Geometry: final body of the model. Coordinates: model frame, mm. Face numbers are marked on the shaded views. A direction names the side the tool comes from. Coordinates: 2 decimals unless noted, no trailing zeros. Write each loop counter-clockwise with the first axis right and the second up, starting at its lowest first coordinate (ties: lowest second). Pieces come first, ordered by that corner, then holes. Notation, with made-up numbers: (33.5, 13) -> (47.5, 13) arc R12 ccw to (47.5, 30) -> close; hole circle Ø10 at (17.25, 54). An arc over 180 degrees is marked (long way). One line per item, written item: value.
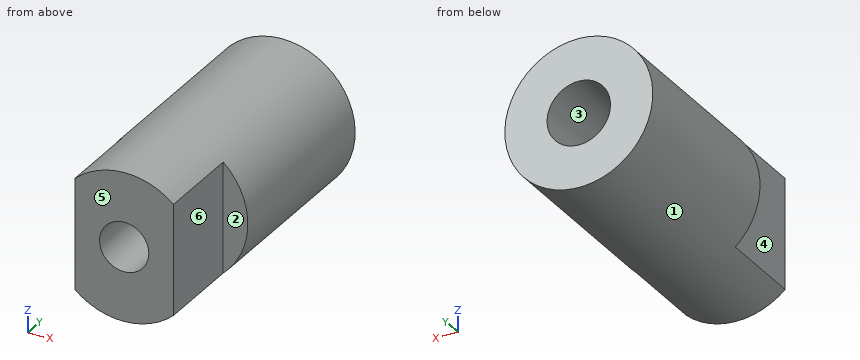
```python
from build123d import *

# Parameters (mm, degrees)
SKETCH1_R                  = 10.5
BOSS_EXTRUDE1_DEPTH        = 40.1
M10X1_0_TAPPED_HOLE1_D     = 9
M10X1_0_TAPPED_HOLE1_DEPTH = 23
M10X1_0_TAPPED_HOLE1_TIP   = 2.703872786
M8X1_0_TAPPED_HOLE1_D      = 7
M8X1_0_TAPPED_HOLE1_DEPTH  = 19
M8X1_0_TAPPED_HOLE1_TIP    = 2.103012167
CUT_EXTRUDE1_DEPTH         = 43.761080435
CUT_EXTRUDE1_DEPTH_BACK    = 43.761080435
SKETCH6_W                  = 3.5
SKETCH6_H                  = 12.7


with BuildPart() as part:
    # Sketch1 → Boss-Extrude1 (new body)
    with BuildSketch(Plane(origin=(0, 0, 0), x_dir=(1, 0, 0), z_dir=(0, 1, 0))):
        with Locations(Location((0, 0, 0), (0, 0, 270))):
            Circle(SKETCH1_R)
    extrude(amount=BOSS_EXTRUDE1_DEPTH)

    # M10x1.0 Tapped Hole1
    with Locations(Plane(origin=(0, 40.1, 0), x_dir=(1, 0, 0), z_dir=(0, 1, 0))):
        with Locations((0, 0)):
            Hole(M10X1_0_TAPPED_HOLE1_D / 2, depth=M10X1_0_TAPPED_HOLE1_DEPTH)
            with Locations((0, 0, -(M10X1_0_TAPPED_HOLE1_DEPTH + M10X1_0_TAPPED_HOLE1_TIP / 2))):  # 118° drill point
                Cone(0, M10X1_0_TAPPED_HOLE1_D / 2, M10X1_0_TAPPED_HOLE1_TIP, mode=Mode.SUBTRACT)

    # M8x1.0 Tapped Hole1
    with Locations(Plane(origin=(0, 0, 0), x_dir=(-1, 0, 0), z_dir=(0, -1, 0))):
        with Locations((0, 0)):
            Hole(M8X1_0_TAPPED_HOLE1_D / 2, depth=M8X1_0_TAPPED_HOLE1_DEPTH)
            with Locations((0, 0, -(M8X1_0_TAPPED_HOLE1_DEPTH + M8X1_0_TAPPED_HOLE1_TIP / 2))):  # 118° drill point
                Cone(0, M8X1_0_TAPPED_HOLE1_D / 2, M8X1_0_TAPPED_HOLE1_TIP, mode=Mode.SUBTRACT)

    # Sketch6 → Cut-Extrude1 (cut, two sides: drawn at the far end of the back side and taken through both)
    with BuildSketch(Plane.XY.offset(-CUT_EXTRUDE1_DEPTH_BACK)):
        with Locations((-8.75, 6.35)):
            Rectangle(SKETCH6_W, SKETCH6_H)
        with Locations((8.75, 6.35)):
            Rectangle(SKETCH6_W, SKETCH6_H)
    extrude(amount=CUT_EXTRUDE1_DEPTH + CUT_EXTRUDE1_DEPTH_BACK, mode=Mode.SUBTRACT)


solid = part.part
```
(1) Section B-B (x = 0). Return the cut outline in (y, z).
Responses:
outline: (0, -10.5) -> (40.1, -10.5) -> (40.1, -4.5) -> (17.1, -4.5) -> (16.5, -3.5) -> (0, -3.5) -> close; (0, 3.5) -> (16.5, 3.5) -> (17.1, 4.5) -> (40.1, 4.5) -> (40.1, 10.5) -> (0, 10.5) -> close
(2) Section C-C (y = 5). Return the cut outline in (x, z), then the cut area to 3 significant figures.
Responses:
outline: (-7, -7.83) arc R10.5 ccw to (7, -7.83) -> (7, 7.83) arc R10.5 ccw to (-7, 7.83) -> close; hole circle Ø7 at (0, 0)
area: 232 mm2
(3) Section D-D (z = -5.5). Return the cut outline in (x, y), then the cut area to 3 significant figures.
Responses:
outline: (-8.94, 12.7) -> (-7, 12.7) -> (-7, 0) -> (7, 0) -> (7, 12.7) -> (8.94, 12.7) -> (8.94, 40.1) -> (-8.94, 40.1) -> close
area: 668 mm2
(4) Pull-direction query (Z, two-part tool) for the marked faces 1, 2 and 3; classes: released by +Z, released by -Z, zero draft, split by the parting line, or undercut.
Responses:
face 1: split by the parting line
face 2: zero draft
face 3: undercut
(5) Section A-A (z = 0). Return the cut outline in (x, y).
Responses:
outline: (-10.5, 12.7) -> (-7, 12.7) -> (-7, 0) -> (-3.5, 0) -> (-3.5, 16.5) -> (-4.5, 17.1) -> (-4.5, 40.1) -> (-10.5, 40.1) -> close; (3.5, 0) -> (7, 0) -> (7, 12.7) -> (10.5, 12.7) -> (10.5, 40.1) -> (4.5, 40.1) -> (4.5, 17.1) -> (3.5, 16.5) -> close
(6) First-contact query: pin 1 (5.5 mm diameter, centred on x = 0, z = 0, fed in from +Y); pin 2 (10 mm diameter, centred on x = -6.5, y = 32, fed in from +Z); pin 3 (1.5 mm diameter, centred on x = -5.5, y = 27.5, fed in from +Z); pin 4 (6.5 mm diameter, centred on y = 5, z = -2, fed in from -X). Flat tips, straight axial feed; report the tip coordinate or a pass-through.
Responses:
pin 1: passes through
pin 2: stops at z = 10.39
pin 3: stops at z = 9.36
pin 4: stops at x = -7
(7) Reachability of the marked faces 4, 5 and 6 from +Z, -Z, +X, -X, +Y, -Y: full face, straight path, thin tool, end or side. Return the list, or none.
Responses:
face 4: +Z, -Z, -X, -Y
face 5: +Z, -Z, +X, -X, -Y
face 6: +Z, -Z, +X, -Y
(8) Line query: line 1 (Z direction, x = 0, y = 11.75); line 2 (X direction, y = 12.5, z = 0.25); line 3 (Z direction, x = 0, y = 29). Output: solid intervals per line, ascending. Write a range as [from, to].
Responses:
line 1: z = [-10.5, -3.5], [3.5, 10.5]
line 2: x = [-7, -3.49], [3.49, 7]
line 3: z = [-10.5, -4.5], [4.5, 10.5]
